The figure shows three views and two pictorial views of one solid part (mm, origin at its lowest corner). Answer the questions. A direction names the side the tool comes from. Give positions to 0.01 mm unless a question says otherwise; leave off trailing zeros. Loops run counter-clockwise (first coordinate to the right, second up) from the corner with the lowest first, then second, coordinate; pieces in that order, holes last. Notation, with made-up numbers: (-19, -39) - (13, -39) arc R17 cw to (13, -22) - close; hole circle Ø9 at (70, -29). An arc over 180 degrees is marked (long way). Use a Markdown table: item, result. Add a question column.
Item 1: Each of these flat-tipped pins is pushed along its axis until it touches: P1, Ø1.2, axis at x = 10, z = 4.5, coming from the -Y side; P2, Ø1.8, axis at y = 2.5, z = 2.5, coming from the -X side; P3, Ø3, axis at x = 16, z = 4.5, coming from the +Y side. Where does it stop, or does it pass through?
Item 2: Consider probe 1 along X at (y, z) = (0.65, 3.8); probe 2 along X at (y, z) = (2.65, 5.5); probe 3 along Y at (x, z) = (10.75, 3.75). Determine where each line is inside the solid, lowest interval first. Write a range as [from, to].
Item 3: Which of the six approach directions +Z, -Z, +X, -X, +Y, -Y give full straight-line access (tool end or side, diameter ignored) to the marked faces 4, 5, 6 and 7?
Item 4: For a pull along X with two mould halves and no side action, classify the marked faces 1, 2 and 3 as +X half, -X half, draft (parallel to the pull), parting line (faces both ways), or undercut.
Item 5: A cutting plane is placed at A-A (y = 3.95). Determine the outline of the cut face in (x, z) (1 decimal), plus the area to 3 significant figures.
Item 6: A cutting plane is placed at B-B (y = 1.25). Determine the outline of the cut face in (x, z), plus the area to 3 significant figures.
Item 7: A cutting plane is placed at C-C (z = 3.8). Give the number of separate pieces and of enclosed holes in the cut face.
Item 8: A cutting plane is placed at D-D (z = 0.5). Determine the outline of the cut face in (x, y).
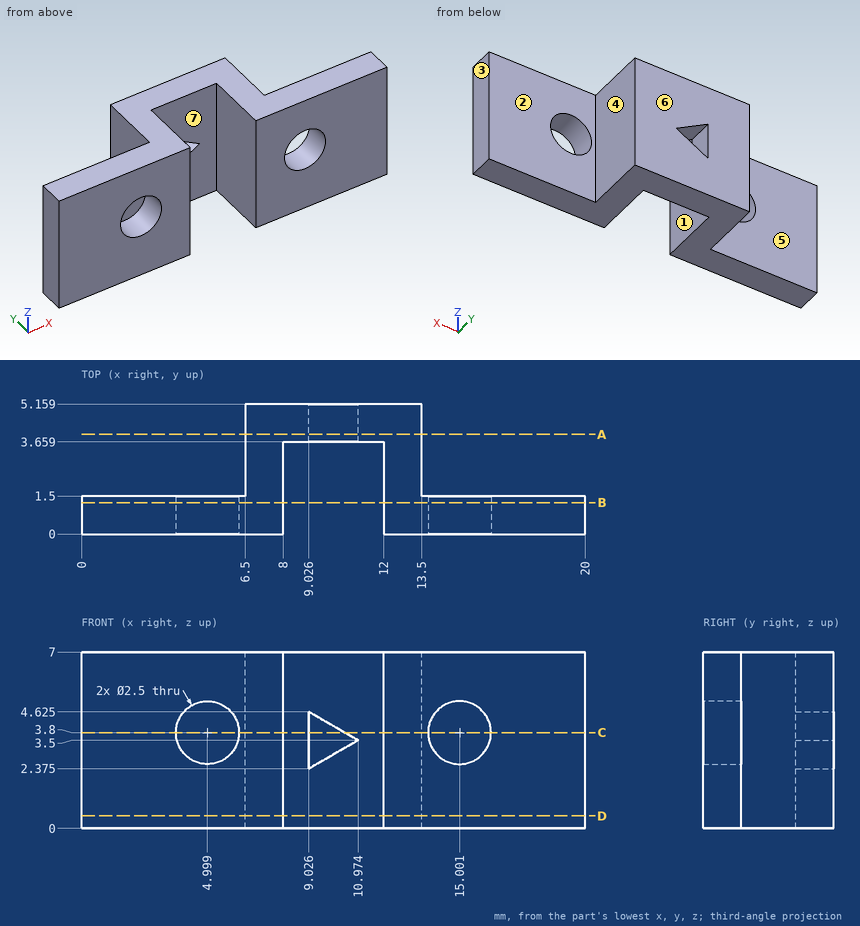
Geometry says:
| question | item | result |
|---|---|---|
| 1 | P1 | y = 3.66 |
| 1 | P2 | x = 6.5 |
| 1 | P3 | y = 1.5 |
| 2 | probe 1 | [0, 3.75], [6.25, 8], [12, 13.75], [16.25, 20] |
| 2 | probe 2 | [6.5, 8], [12, 13.5] |
| 2 | probe 3 | [3.66, 5.16] |
| 3 | face 4 | +Z, -Z, +X, +Y |
| 3 | face 5 | +Z, -Z, -X, +Y |
| 3 | face 6 | +Z, -Z, +X, -X, +Y |
| 3 | face 7 | +Z, -Z, -Y |
| 4 | face 1 | undercut |
| 4 | face 2 | draft |
| 4 | face 3 | +X half |
| 5 | outline | (6.5, 0) - (13.5, 0) - (13.5, 7) - (6.5, 7) - close; hole (9, 2.4) - (11, 3.5) - (9, 4.6) - close |
| 5 | area | 46.8 mm² |
| 6 | outline | (0, 0) - (8, 0) - (8, 7) - (0, 7) - close; (12, 0) - (20, 0) - (20, 7) - (12, 7) - close; hole circle Ø2.5 at (5, 3.8); hole circle Ø2.5 at (15, 3.8) |
| 6 | area | 102 mm² |
| 7 | separate pieces | 4 |
| 7 | enclosed holes | 0 |
| 8 | outline | (0, 0) - (8, 0) - (8, 3.66) - (12, 3.66) - (12, 0) - (20, 0) - (20, 1.5) - (13.5, 1.5) - (13.5, 5.16) - (6.5, 5.16) - (6.5, 1.5) - (0, 1.5) - close |
